Part model, mm, in its own coordinate system. A direction names the side the tool comes from. Round coordinates to 2 decimals unless told otherwise and drop trailing zeros. Loops run counter-clockwise (first coordinate to the right, second up) from the corner with the lowest first, then second, coordinate; pieces in that order, holes last. Notation, with made-up numbers: (78, 53.25) - (110, 53.25) arc R31 ccw to (110, 82.25) - close; hole circle Ø3 at (-31.5, 62.25). An arc over 180 degrees is marked (long way). Put each result on its own line as item: value.
from build123d import *

# Parameters (mm, degrees)
F0_W     = 33.02
F0_H     = 44.45
F0_R     = 1.75
F1_DEPTH = 2
F2_SIZE  = 7.62
F3_R     = 6.5
F4_DEPTH = 1.27


with BuildPart() as f1:
    # F0 (on Top) → F1 (new body)
    with BuildSketch(Plane.XY):
        with Locations((16.51, 0)):
            Rectangle(F0_W, F0_H)
        with Locations((6.35, -17.78)):
            Circle(F0_R, mode=Mode.SUBTRACT)
        with Locations((22.86, -17.78)):
            Circle(F0_R, mode=Mode.SUBTRACT)
        with BuildLine():
            ThreePointArc((13.1675, 4.580534), (15.461886, 2.782821), (16.329, 0))
            ThreePointArc((16.329, 0), (15.461886, -2.782821), (13.1675, -4.580534))
            Line((13.1675, -4.580534), (13.1675, -13.97))
            Line((13.1675, -13.97), (11.43, -13.97))
            Line((11.43, -13.97), (9.6925, -13.97))
            Line((9.6925, -13.97), (9.6925, -4.580534))
            ThreePointArc((9.6925, -4.580534), (6.531, 0), (9.6925, 4.580534))
            Line((9.6925, 4.580534), (9.6925, 13.97))
            Line((9.6925, 13.97), (11.43, 13.97))
            Line((11.43, 13.97), (13.1675, 13.97))
            Line((13.1675, 13.97), (13.1675, 4.580534))
        make_face(mode=Mode.SUBTRACT)
        with Locations((6.35, 17.78)):
            Circle(F0_R, mode=Mode.SUBTRACT)
        with Locations((22.86, 17.78)):
            Circle(F0_R, mode=Mode.SUBTRACT)
    extrude(amount=F1_DEPTH)

    # F2
    f2_edges = [f1.edges().sort_by_distance(p)[0] for p in [
        (33.02, -22.225, 1),
        (33.02, 22.225, 1),
    ]]
    chamfer(f2_edges, length=F2_SIZE)

    # F3 (on face) → F4 (cut)
    with BuildSketch(Plane.XY.offset(2)):
        with Locations((11.43, 0)):
            Circle(F3_R)
    extrude(amount=-F4_DEPTH, mode=Mode.SUBTRACT)


solid = f1.part
1. Probe line 1 along Y through (x, z) = (22.86, 0.7) (3 decimals); line 2 along X through (y, z) = (10, 1); line 3 along Y through (x, z) = (12.5, 0.4) (3 decimals). List the from-to ranges inside material, lowest first. Write a range as [from, to].
A:
line 1: y = [-22.225, -19.53], [-16.03, 16.03], [19.53, 22.225]
line 2: x = [0, 9.69], [13.17, 33.02]
line 3: y = [-22.225, -13.97], [13.97, 22.225]
2. Tool access for faces 1 (the cylindrical face through (6.53, -0.08, 0.36)), 2 (the cylindrical face through (17.93, -0.12, 1.37)), 3 (the flat face through (20, 0, 2)): list every direction of +Z, -Z, +X, -X, +Y, -Y with a clear straight run to the whole face (end or side of a thin tool).
A:
face 1: +Z, -Z
face 2: +Z
face 3: +Z, +X, -X, +Y, -Y
3. Band-saw the part on C-C (y = 17.78). List the corners of the cut face in (x, z) (3 decimals), plus the area to 3 significant figures.
A:
outline: (0, 0) - (4.6, 0) - (4.6, 2) - (0, 2) - close; (8.1, 0) - (21.11, 0) - (21.11, 2) - (8.1, 2) - close; (24.61, 0) - (29.845, 0) - (29.845, 2) - (24.61, 2) - close
area: 45.7 mm²
4. Band-saw the part on A-A (x = 22.86). List the corners of the cut face in (y, z) (3 decimals), plus the area to 3 significant figures.
A:
outline: (-22.225, 0) - (-19.53, 0) - (-19.53, 2) - (-22.225, 2) - close; (-16.03, 0) - (16.03, 0) - (16.03, 2) - (-16.03, 2) - close; (19.53, 0) - (22.225, 0) - (22.225, 2) - (19.53, 2) - close
area: 74.9 mm²
5. Pin check, flat tips, straight feed: P1, Ø2, axis at x = 22.86, y = -17.78, coming from the +Z side; P2, Ø2.5, axis at x = 7.5, y = -2, coming from the +Z side. Stop position of each tip, or through.
A:
P1: passes through
P2: stops at z = 0.73
6. Band-saw the part on D-D (x = 10.5). List the corners of the cut face in (y, z) (3 decimals), plus the area to 3 significant figures.
A:
outline: (-22.225, 0) - (-13.97, 0) - (-13.97, 2) - (-22.225, 2) - close; (13.97, 0) - (22.225, 0) - (22.225, 2) - (13.97, 2) - close
area: 33.0 mm²
7. Band-saw the part on B-B (z = 0.3). Give the number of separate pieces and of enclosed holes in the cut face, plus the area to 3 significant figures.
A:
separate pieces: 1
enclosed holes: 5
area: 1,230 mm²
8. Two-plate mould, pull along X, no slides. Class faces 4 (the flat face through (17, 0, 0.73)), 5 (the flat face through (13, 22.225, 1)), 6 (the flat face through (29.263, 18.362, 0.986)): pulls with the +X half, pulls with the -X half, needs draft (parallel to the pull), parting line crosses it, or undercut.
A:
face 4: undercut
face 5: needs draft
face 6: pulls with the +X half
